Autodesk Inventor part; units mm, degrees
ref_plane "YZ Plane" through (0, 0, 0) normal (1, 0, 0) x (0, 1, 0)
ref_plane "XZ Plane" through (0, 0, 0) normal (0, 1, 0) x (-1, 0, 0)
ref_plane "XY Plane" through (0, 0, 0) normal (0, 0, 1) x (1, 0, 0)
sketch "Esboço1" plane through (0, 0, 0) normal (0, 1, 0) x (-1, 0, 0)
  circle A0 centre (0, 0) radius 3
  line L0 (-2.8868, -5) -> (-5.7735, 0)
  line L1 (-5.7735, 0) -> (-2.8868, 5)
  line L2 (-2.8868, 5) -> (2.8868, 5)
  line L3 (2.8868, 5) -> (5.7735, 0)
  line L4 (5.7735, 0) -> (2.8868, -5)
  line L5 (2.8868, -5) -> (-2.8868, -5)
  dimension "d0" = 6
extrude "Extrusão1" add sketch "Esboço1" along normal blind 5
sketch "Esboço2" plane through (0, 0, 0) normal (1, 0, 0) x (0, 1, 0)
  point P0 (0, 0)
chamfer "Chanfro1" distance 0.5 angle 45 2 edges at (3, 0, 0) (3, 5, 0)
sketch "Esboço5" plane through (0, 0, 0) normal (0, -1, 0) x (1, 0, 0)
  circle A0 centre (0, 0) radius 5
extrude "Extrusão2" cut sketch "Esboço5" against normal through all draft 45 keep common part
sketch "Esboço6" plane through (0, 5, 0) normal (0, 1, 0) x (1, 0, 0)
  circle A0 centre (0, 0) radius 5
extrude "Extrusão3" cut sketch "Esboço6" against normal through all draft 45 keep common part
sketch "Esboço7" plane through (0, 5, 0) normal (0, 1, 0) x (1, 0, 0)
  circle A0 centre (0, 0) radius 3.5
extrude "Extrusão4" add sketch "Esboço7" against normal blind 5
sketch "Esboço8" plane through (0, 5, 0) normal (0, 1, 0) x (1, 0, 0)
  circle A0 centre (0, 0) radius 3.175
  dimension "d16" = 6.35
extrude "Extrusão5" add sketch "Esboço8" along normal blind 16
fillet "Arredondamento2" radius 0.4 1 edges at (-3.175, 5, 0)
chamfer "Chanfro3" distance 0.5 angle 45 1 edges at (-3.175, 21, 0)
thread "Rosca3"
properties part number "porca m6" material "Aço inoxidável"
Model file for the job. Use its own axes, mm. A direction names the side the tool comes from. Give positions to 0.01 mm unless a question says otherwise; leave off trailing zeros. Order: outer loops, then holes, each group sorted by start corner. A loop starts at its lowest first (then second) coordinate and runs counter-clockwise, first axis right, second up. Notation, with made-up numbers: M 39.5,3 L 44.5,3 A15 ccw 44.5,27 Z; hole C 85,60 d2. An arc over 180 degrees is marked long. Write item = value, one per line.
Q1. Drill centre lines: line 1 (Y direction, x = -2, z = -3); line 2 (Z direction, x = 1, y = 9); line 3 (Y direction, x = -2.25, z = -1.5). Where is each one in solid material? Low to high. Write a range as [from, to].
Derived:
line_1 = [0, 5]
line_2 = [-3.01, 3.01]
line_3 = [0, 20.97]
Q2. Tool access for faces 1 (the conical face through (-2.583, 4.812, 4.499)), 2 (the flat face through (3.3, 5, 2.2)): list every direction of +Z, -Z, +X, -X, +Y, -Y with a clear straight run to the whole face (end or side of a thin tool).
Derived:
face_1 = +Z, -X, +Y
face_2 = +Y
Q3. Flat gauge pins, fed straight in: pin 1 (1.5 mm diameter, centred on x = -2.5, z = -2.5, fed in from +Y); pin 2 (1 mm diameter, centred on x = -2, y = 9.5, fed in from +Z); pin 3 (2 mm diameter, centred on y = 4.5, z = -1.5, fed in from +X). Where does each tip first touch, or does it go through?
Derived:
pin_1 = 20.89
pin_2 = 2.8
pin_3 = 5.48
Q4. Cut at B-B, the plane y = 8. List the corners of the cut face in (x, z) (3 decimals).
Derived:
outline = C 0,0 d6.35
Q5. Cut at A-A, the plane y = 3.25. List the corners of the cut face in (x, z), then the cut area to 3 significant figures.
Derived:
outline = M -5.77,0 L -2.89,-5 L 2.89,-5 L 5.77,0 L 2.89,5 L -2.89,5 Z
area = 86.6 mm2
